from build123d import *

# Parameters (mm, degrees)
F0_W     = 254
F0_H     = 304.8
F1_DEPTH = 152.4
F2_W     = 12.7
F2_H     = 25.4
F3_DEPTH = 25.4
F4_R     = 12.7
F4_R_2   = 11.43
F4_W     = 28.194
F4_H     = 46.99
F4_W_2   = 14.986
F4_H_2   = 22.86
F4_R_3   = 9.525
F5_DEPTH = 25.4


with BuildPart() as f1:
    # F0 (on Front) → F1 (new body)
    with BuildSketch(Plane.XZ):
        Rectangle(F0_W, F0_H)
    extrude(amount=F1_DEPTH)

    # F2 (on face) → F3 (join)
    with BuildSketch(Plane.YZ.offset(127)):
        with Locations((-120.65, 95.25)):
            Rectangle(F2_W, F2_H)
        with Locations((-120.65, -95.25)):
            Rectangle(F2_W, F2_H)
    extrude(amount=F3_DEPTH)

    # F4 (on face) → F5 (cut)
    with BuildSketch(Plane.YZ.offset(127)):
        with Locations((-101.6, -5.08)):
            Circle(F4_R)
        with Locations((-63.5, -5.08)):
            Circle(F4_R)
        with Locations((-25.4, -5.08)):
            Circle(F4_R)
        with Locations((-101.6, -55.88)):
            Circle(F4_R_2)
        with Locations((-63.5, -55.88)):
            Circle(F4_R_2)
        with Locations((-25.4, -55.88)):
            Circle(F4_R_2)
        with Locations((-26.797, -116.205)):
            Rectangle(F4_W, F4_H)
        with Locations((-25.4, 45.72)):
            Rectangle(F4_W_2, F4_H_2)
        with Locations((-101.6, 45.72)):
            Circle(F4_R_3)
        with Locations((-63.5, 45.72)):
            Circle(F4_R_3)
    extrude(amount=-F5_DEPTH, mode=Mode.SUBTRACT)


solid = f1.part
Verification items for the finished model (mm, model axes). A direction names the side the tool comes from. Round coordinates to 2 decimals unless told otherwise and drop trailing zeros. Loops run counter-clockwise (first coordinate to the right, second up) from the corner with the lowest first, then second, coordinate; pieces in that order, holes last. Notation, with made-up numbers: (-33.5, 14.25) - (-15.5, 14.25) arc R18 cw to (-15.5, 31.25) - close; hole circle Ø9 at (14.25, 13). An arc over 180 degrees is marked (long way). Use a Markdown table: item, result. Add a question column.
1. Section check D-D, the plane y = -101.6. Record the boundary of the cut face in (x, z) (3 decimals), plus the area to 3 significant figures.
2. Access from +Z, -Z, +X, -X, +Y, -Y to the whole of each face (thin tool, end or side, straight path). Record for faces 5 (the face through (140, -121, 82.55)), 6 (the face through (140, -114.3, -95)), 7 (the face through (152.4, -121, -95)), 8 (the face through (101.6, -64, -56)).
3. Section check A-A, the plane y = -25.4. Record the boundary of the cut face in (x, z), plus the area to 3 significant figures.
4. Section check B-B, the plane z = -55.88. Record the boundary of the cut face in (x, y), plus the area to 3 significant figures.
5. Section check C-C, the plane z = -102. Record the boundary of the cut face in (x, y).
6. Release check for a two-part mould opening along Z. For faces 1 (the face through (-2, -152.4, 2)), 2 (the face through (-2, -75, -152.4)), 3 (the face through (114.478, -89.486, -1.265)), 4 (the face through (-2, -75, 152.4)) record: released by +Z, released by -Z, zero draft, split by the parting line, or undercut.
7. Gauge pin test, flat ends, axial feed: pin 1 (23 mm diameter, centred on y = -101.6, z = -5.08, fed in from +X); pin 2 (10 mm diameter, centred on x = 144.5, y = -121, fed in from -Z); pin 3 (20.5 mm diameter, centred on y = -98.5, z = -7, fed in from +X). Record the tip position at first contact, or that the pin passes through.
8. Thickness scan on probe 1 along Z at (x, y) = (111, -63); probe 2 along Y at (x, z) = (109, -55); probe 3 along Y at (x, z) = (119, -5). Record the ranges inside material, lowest first. Write a range as [from, to].
Checks:
| question | item | result |
|---|---|---|
| 1 | outline | (-127, -152.4) - (127, -152.4) - (127, -67.31) - (101.6, -67.31) - (101.6, -44.45) - (127, -44.45) - (127, -17.78) - (101.6, -17.78) - (101.6, 7.62) - (127, 7.62) - (127, 36.195) - (101.6, 36.195) - (101.6, 55.245) - (127, 55.245) - (127, 152.4) - (-127, 152.4) - close |
| 1 | area | 75,700 mm^2 |
| 2 | face 5 | +X, +Y, -Y |
| 2 | face 6 | +Z, -Z, +X, +Y |
| 2 | face 7 | +Z, -Z, +X, +Y, -Y |
| 2 | face 8 | +X |
| 3 | outline | (-127, -152.4) - (127, -152.4) - (127, -139.7) - (101.6, -139.7) - (101.6, -92.71) - (127, -92.71) - (127, -67.31) - (101.6, -67.31) - (101.6, -44.45) - (127, -44.45) - (127, -17.78) - (101.6, -17.78) - (101.6, 7.62) - (127, 7.62) - (127, 34.29) - (101.6, 34.29) - (101.6, 57.15) - (127, 57.15) - (127, 152.4) - (-127, 152.4) - close |
| 3 | area | 74,400 mm^2 |
| 4 | outline | (-127, -152.4) - (127, -152.4) - (127, -113.03) - (101.6, -113.03) - (101.6, -90.17) - (127, -90.17) - (127, -74.93) - (101.6, -74.93) - (101.6, -52.07) - (127, -52.07) - (127, -36.83) - (101.6, -36.83) - (101.6, -13.97) - (127, -13.97) - (127, 0) - (-127, 0) - close |
| 4 | area | 37,000 mm^2 |
| 5 | outline | (-127, -152.4) - (127, -152.4) - (127, -127) - (152.4, -127) - (152.4, -114.3) - (127, -114.3) - (127, -40.89) - (101.6, -40.89) - (101.6, -12.7) - (127, -12.7) - (127, 0) - (-127, 0) - close |
| 6 | face 1 | zero draft |
| 6 | face 2 | released by -Z |
| 6 | face 3 | undercut |
| 6 | face 4 | released by +Z |
| 7 | pin 1 | stops at x = 101.6 |
| 7 | pin 2 | stops at z = -107.95 |
| 7 | pin 3 | stops at x = 127 |
| 8 | probe 1 | z = [-152.4, -67.3], [-44.46, -17.77], [7.61, 36.21], [55.23, 152.4] |
| 8 | probe 2 | y = [-152.4, -113], [-90.2, -74.9], [-52.1, -36.8], [-14, 0] |
| 8 | probe 3 | y = [-152.4, -114.3], [-88.9, -76.2], [-50.8, -38.1], [-12.7, 0] |
